Design review of the part built by this model. Coordinates are the model's own, in mm. A direction names the side the tool comes from. Give positions to 0.01 mm unless a question says otherwise; leave off trailing zeros. Order: outer loops, then holes, each group sorted by start corner. A loop starts at its lowest first (then second) coordinate and runs counter-clockwise, first axis right, second up. Notation, with made-up numbers: M -20,43 L 33,43 A34 cw 33,81 Z; hole C -27,5 d6. An arc over 180 degrees is marked long. Put each result on its own line as item: value. Start each with the question number.
from build123d import *

# Parameters (mm, degrees)
CROQUIS1_W                 = 50
CROQUIS1_H                 = 50
SALIENTE_EXTRUIR1_DEPTH    = 50
CORTAR_EXTRUIR1_DEPTH      = 50
CORTAR_EXTRUIR2_DEPTH      = 25
CORTAR_EXTRUIR2_DEPTH_BACK = 25
VACIADO1_T                 = -2.5
CORTAR_EXTRUIR3_DEPTH      = 2.5
CORTAR_EXTRUIR4_DEPTH      = 2.5
CORTAR_EXTRUIR5_DEPTH      = 2.5
CORTAR_EXTRUIR6_DEPTH      = 2.5


with BuildPart() as part:
    # Croquis1 → Saliente-Extruir1 (new body)
    with BuildSketch(Plane(origin=(0, 0, 0), x_dir=(1, 0, 0), z_dir=(0, 1, 0))):
        Rectangle(CROQUIS1_W, CROQUIS1_H)
    extrude(amount=SALIENTE_EXTRUIR1_DEPTH)

    # Croquis2 → Cortar-Extruir1 (cut)
    with BuildSketch(Plane.ZY.offset(25)):
        Polygon((-25, 0), (0, 50), (-25, 50), align=None)
        Polygon((0, 50), (25, 0), (25, 50), align=None)
    extrude(amount=-CORTAR_EXTRUIR1_DEPTH, mode=Mode.SUBTRACT)

    # Croquis4 → Cortar-Extruir2 (cut, two sides)
    with BuildSketch(Plane(origin=(0, 0, 0), x_dir=(-1, 0, 0), z_dir=(0, 0, -1))) as cortar_extruir2_sk:
        Polygon((-25, 50), (-25, 0), (0, 50), align=None)
        Polygon((25, 50), (0, 50), (25, 0), align=None)
    extrude(amount=CORTAR_EXTRUIR2_DEPTH, mode=Mode.SUBTRACT)
    extrude(cortar_extruir2_sk.sketch, amount=-CORTAR_EXTRUIR2_DEPTH_BACK, mode=Mode.SUBTRACT)

    # Vaciado1
    vaciado1_openings = [part.faces().sort_by_distance(p)[0] for p in [
        (0, 0, 0),
    ]]
    offset(amount=VACIADO1_T, openings=vaciado1_openings, kind=Kind.INTERSECTION)

    # Croquis6 → Cortar-Extruir3 (cut)
    with BuildSketch(Plane(origin=(0, 10, -20), x_dir=(-1, 0, 0), z_dir=(0, 0.447213595, -0.894427191))):
        Polygon((0, 38.597635193), (-21.143353224, -8.680339887), (21.143353224, -8.680339887), align=None)
    extrude(amount=-CORTAR_EXTRUIR3_DEPTH, mode=Mode.SUBTRACT)

    # Croquis7 → Cortar-Extruir4 (cut)
    with BuildSketch(Plane(origin=(-20, 10, 0), x_dir=(0, 0, 1), z_dir=(-0.894427191, 0.447213595, 0))):
        Polygon((-21.143353224, -8.680339887), (21.143353224, -8.680339887), (0, 38.597635193), align=None)
    extrude(amount=-CORTAR_EXTRUIR4_DEPTH, mode=Mode.SUBTRACT)

    # Croquis8 → Cortar-Extruir5 (cut)
    with BuildSketch(Plane(origin=(0, 10, 20), x_dir=(1, 0, 0), z_dir=(0, 0.447213595, 0.894427191))):
        Polygon((-21.143353224, -8.680339887), (21.143353224, -8.680339887), (0, 38.597635193), align=None)
    extrude(amount=-CORTAR_EXTRUIR5_DEPTH, mode=Mode.SUBTRACT)

    # Croquis9 → Cortar-Extruir6 (cut)
    with BuildSketch(Plane(origin=(20, 10, 0), x_dir=(0, 0, -1), z_dir=(0.894427191, 0.447213595, 0))):
        Polygon((21.143353224, -8.680339887), (0, 38.597635193), (-21.143353224, -8.680339887), align=None)
    extrude(amount=-CORTAR_EXTRUIR6_DEPTH, mode=Mode.SUBTRACT)


solid = part.part
1. Insertion check: pin 1 (1 mm diameter, centred on y = 38.5, z = -4, fed in from -X); pin 2 (4 mm diameter, centred on x = -3.5, y = 42, fed in from +Z); pin 3 (8 mm diameter, centred on y = 16.5, z = 14, fed in from +X). Each pin has a flat end and moves straight along its axis. Give the tip position at first contact, or say it passes through.
2. To check wall thickness, follow probe 1 along Z at (x, y) = (14.5, 18.5); probe 2 along Z at (x, y) = (-13, 21); probe 3 along Y at (x, z) = (-22, 7). State the ranges of each line that lie inside material, in increasing order.
3. The part is to be moulded in two halves that separate along X. For faces 3 (the flat face through (-13.37, 23.26, 10.99)), 4 (the flat face through (-10.72, 22.53, -12.36)), 5 (the flat face through (10.99, 23.26, 13.37)), say which applies: +X half, -X half, draft (parallel to the pull), parting line (faces both ways), or undercut.
4. Consider section A-A on x = 17.5. Give the boundary of the cut face in (y, z).
5. Consider section C-C on z = -11.5. Give the boundary of the cut face in (x, y), then the cut area to 3 significant figures.
6. Consider section B-B on y = 11. Give the boundary of the cut face in (x, z).
7. Machinability: for faces 1 (the flat face through (13.5, 23, -11.2)), 2 (the flat face through (-3.393, 0.719, -21.846)), which of the approach directions +Z, -Z, +X, -X, +Y, -Y give a long, thin tool a straight path to every point of the face, cutting with its end or side? Answer none if there is none.
Returned:
1. pin 1: stops at x = -6
1. pin 2: stops at z = 5
1. pin 3: stops at x = 18.54
2. probe 1: z = -15.75 to -12.76, 12.76 to 15.75
2. probe 2: z = -14.5 to -11.46, 11.46 to 14.5
2. probe 3: y = 0.41 to 1.3
3. face 3: -X half
3. face 4: undercut
3. face 5: draft
4. outline: M 0,-25 L 2.24,-23.88 L 1.12,-21.65 L 0,-22.2 Z; M 0,22.2 L 1.12,21.65 L 2.24,23.88 L 0,25 Z; M 8.4,-18 L 9.52,-20.24 L 15,-17.5 L 15,-14.76 L 9.41,-17 L 9.41,-17.5 Z; M 8.4,18 L 9.41,17.5 L 9.41,17 L 15,14.76 L 15,17.5 L 9.52,20.24 Z
5. outline: M -25,0 L -22.2,0 L -21.65,1.12 L -23.88,2.24 Z; M -14.24,21.52 L -12,20.4 L -11.5,21.41 L -11,21.41 L -8.76,27 L -11.5,27 Z; M 8.76,27 L 11,21.41 L 11.5,21.41 L 12,20.4 L 14.24,21.52 L 11.5,27 Z; M 21.65,1.12 L 22.2,0 L 25,0 L 23.88,2.24 Z
5. area: 45.6 mm2
6. outline: M -19.5,-19.5 L -16.76,-19.5 L -16.2,-16.7 L -16.7,-16.7 L -16.7,-16.2 L -19.5,-16.76 Z; M -19.5,16.76 L -16.7,16.2 L -16.7,16.7 L -16.2,16.7 L -16.76,19.5 L -19.5,19.5 Z; M 16.2,-16.7 L 16.76,-19.5 L 19.5,-19.5 L 19.5,-16.76 L 16.7,-16.2 L 16.7,-16.7 Z; M 16.2,16.7 L 16.7,16.7 L 16.7,16.2 L 19.5,16.76 L 19.5,19.5 L 16.76,19.5 Z
7. face 1: +Z, -Z, +X, +Y
7. face 2: -Y
